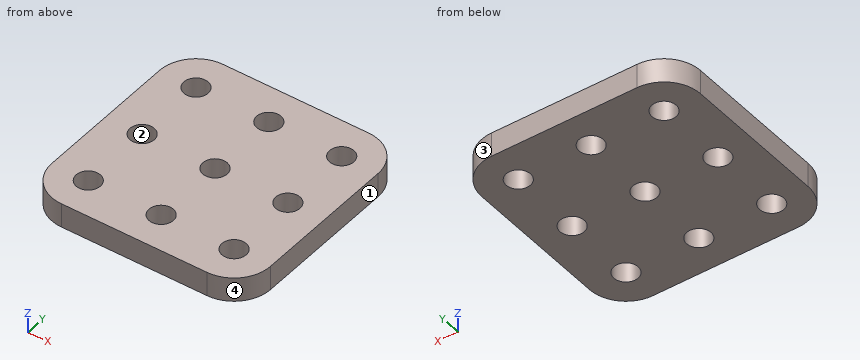
from build123d import *

# Parameters (mm, degrees)
MODEL_R                 = 1.5
SALIENTE_EXTRUIR1_DEPTH = 3


with BuildPart() as part:
    # Model → Saliente-Extruir1 (new body)
    with BuildSketch(Plane.XY):
        with BuildLine():
            Line((-105.943383637, 101.056539338), (-105.943383637, 83.056539338))
            ThreePointArc((-105.943383637, 83.056539338), (-104.625364152, 79.874558823), (-101.443383637, 78.556539338))
            Line((-101.443383637, 78.556539338), (-83.443383637, 78.556539338))
            ThreePointArc((-83.443383637, 78.556539338), (-80.261403122, 79.874558823), (-78.943383637, 83.056539338))
            Line((-78.943383637, 83.056539338), (-78.943383637, 101.056539338))
            ThreePointArc((-78.943383637, 101.056539338), (-80.261403122, 104.238519853), (-83.443383637, 105.556539338))
            Line((-83.443383637, 105.556539338), (-101.443383637, 105.556539338))
            ThreePointArc((-101.443383637, 105.556539338), (-104.625364152, 104.238519853), (-105.943383637, 101.056539338))
        make_face()
        with Locations((-101.443383637, 101.056539338)):
            Circle(MODEL_R, mode=Mode.SUBTRACT)
        with Locations((-92.443383637, 101.056539338)):
            Circle(MODEL_R, mode=Mode.SUBTRACT)
        with Locations((-83.443383637, 101.056539338)):
            Circle(MODEL_R, mode=Mode.SUBTRACT)
        with Locations((-101.443383637, 92.056539338)):
            Circle(MODEL_R, mode=Mode.SUBTRACT)
        with Locations((-92.443383637, 92.056539338)):
            Circle(MODEL_R, mode=Mode.SUBTRACT)
        with Locations((-83.443383637, 92.056539338)):
            Circle(MODEL_R, mode=Mode.SUBTRACT)
        with Locations((-101.443383637, 83.056539338)):
            Circle(MODEL_R, mode=Mode.SUBTRACT)
        with Locations((-92.443383637, 83.056539338)):
            Circle(MODEL_R, mode=Mode.SUBTRACT)
        with Locations((-83.443383637, 83.056539338)):
            Circle(MODEL_R, mode=Mode.SUBTRACT)
    extrude(amount=SALIENTE_EXTRUIR1_DEPTH)


solid = part.part
The listing builds one solid part. Answer for the finished solid, in the listing's coordinates (mm). Face numbers are marked on the shaded views. Give positions to 0.01 mm unless a question says otherwise; leave off trailing zeros. Write each loop counter-clockwise with the first axis right and the second up, starting at its lowest first coordinate (ties: lowest second). Pieces come first, ordered by that corner, then holes.
1) Section B-B (x = -84) is taken. Write down the section's boundary in (y, z).
2) Find the intervals of material crossed by L1, parallel to X at y = 101, z = 2.8; L2, parallel to Y at x = -92, z = 1.1; L3, parallel to Y at x = -93.75, z = 1.4, in increasing order.
3) Section C-C (z = 0.5) is taken. Count the separate pieces of the cut face and the enclosed holes in it, and give its area (3 significant figures).
4) Section A-A (y = 91) is taken. Write down the section's boundary in (x, z), and give its area (3 significant figures).
5) For a pull along Y with two mould halves and no side action, classify the marked faces 1, 2, 3 and 4 as pulls with the +Y half, pulls with the -Y half, needs draft (parallel to the pull), parting line crosses it, or undercut.
6) Section D-D (x = -80.75) is taken. Write down the section's boundary in (y, z), and give its area (3 significant figures).
Response:
1. outline: (78.56, 0) - (81.66, 0) - (81.66, 3) - (78.56, 3) - close; (84.45, 0) - (90.66, 0) - (90.66, 3) - (84.45, 3) - close; (93.45, 0) - (99.66, 0) - (99.66, 3) - (93.45, 3) - close; (102.45, 0) - (105.56, 0) - (105.56, 3) - (102.45, 3) - close
2. L1: x = -105.94 to -102.94, -99.94 to -93.94, -90.94 to -84.94, -81.94 to -78.94
2. L2: y = 78.56 to 81.62, 84.49 to 90.62, 93.49 to 99.62, 102.49 to 105.56
2. L3: y = 78.56 to 82.32, 83.79 to 91.32, 92.79 to 100.32, 101.79 to 105.56
3. separate pieces: 1
3. enclosed holes: 9
3. area: 648 mm2
4. outline: (-105.94, 0) - (-102.51, 0) - (-102.51, 3) - (-105.94, 3) - close; (-100.38, 0) - (-93.51, 0) - (-93.51, 3) - (-100.38, 3) - close; (-91.38, 0) - (-84.51, 0) - (-84.51, 3) - (-91.38, 3) - close; (-82.38, 0) - (-78.94, 0) - (-78.94, 3) - (-82.38, 3) - close
4. area: 61.8 mm2
5. face 1: needs draft
5. face 2: undercut
5. face 3: pulls with the +Y half
5. face 4: pulls with the -Y half
6. outline: (79.45, 0) - (104.66, 0) - (104.66, 3) - (79.45, 3) - close
6. area: 75.6 mm2
